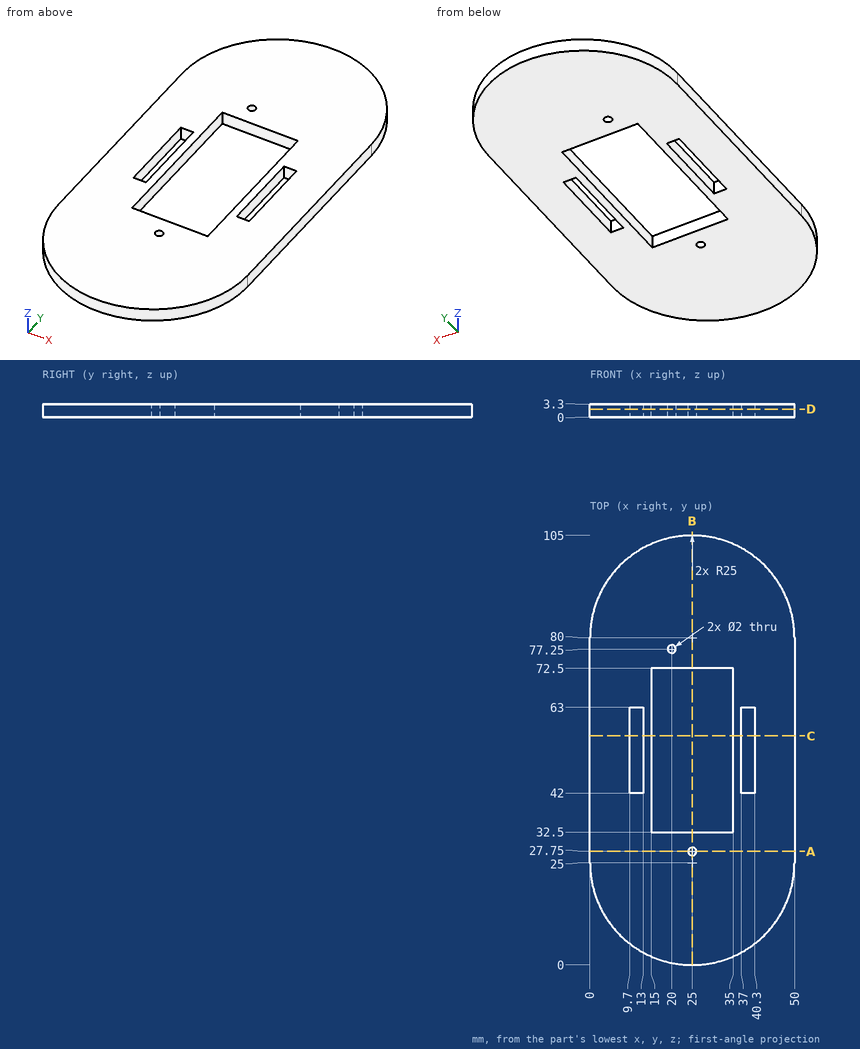
Geometry: see drawing. Coordinates: mm, zero at the bounding-box minimum. Give positions to 0.01 mm unless a question says otherwise; leave off trailing zeros. Order: outer loops, then holes, each group sorted by start corner. A loop starts at its lowest first (then second) coordinate and runs counter-clockwise, first axis right, second up. Notation, with made-up numbers: (-31.75, -5) -> (10.25, -5) arc R21 cw to (10.25, 15) -> close; hole circle Ø9 at (62.25, 85). An arc over 180 degrees is marked (long way). Write each question's results on one line, items separated by ' | '. Start each with the question number.
1) Section B-B (x = 25). Return loops of the section in (y, z).
2) Section A-A (y = 27.75). Return loops of the section in (x, z), then the cut area to 3 significant figures.
3) Section D-D (z = 2.05). Return loops of the section in (x, y).
4) Line query: line 1 (Y direction, x = 20, z = 2.5); line 2 (X direction, y = 57, z = 1.2); line 3 (Y direction, x = 25, z = 3.1). Output: solid intervals per line, ascending. Write a range as from..to.
5) Section C-C (y = 56). Return loops of the section in (x, z), then the cut area to 3 significant figures.
6) First-contact query: pin 1 (1.6 mm diameter, centred on x = 12, z = 1, fed in from +Y); pin 2 (1 mm diameter, centred on x = 11, z = 1, fed in from -Y); pin 3 (1.6 mm diameter, centred on x = 22.5, z = 1.5, fed in from -Y). Flat tips, straight axial feed; report the tip coordinate or a pass-through.
Calculated:
1) outline: (0, 0) -> (26.75, 0) -> (26.75, 3.3) -> (0, 3.3) -> close; (28.75, 0) -> (32.5, 0) -> (32.5, 3.3) -> (28.75, 3.3) -> close; (72.5, 0) -> (105, 0) -> (105, 3.3) -> (72.5, 3.3) -> close
2) outline: (0, 0) -> (24, 0) -> (24, 3.3) -> (0, 3.3) -> close; (26, 0) -> (50, 0) -> (50, 3.3) -> (26, 3.3) -> close | area: 158 mm2
3) outline: (0, 25) arc R25 ccw to (50, 25) -> (50, 80) arc R25 ccw to (0, 80) -> close; hole (9.7, 42) -> (13, 42) -> (13, 63) -> (9.7, 63) -> close; hole (15, 32.5) -> (35, 32.5) -> (35, 72.5) -> (15, 72.5) -> close; hole circle Ø2 at (20, 77.25); hole circle Ø2 at (25, 27.75); hole (37, 42) -> (40.3, 42) -> (40.3, 63) -> (37, 63) -> close
4) line 1: 0.51..32.5, 72.5..76.25, 78.25..104.49 | line 2: 0..9.7, 13..15, 35..37, 40.3..50 | line 3: 0..26.75, 28.75..32.5, 72.5..105
5) outline: (0, 0) -> (9.7, 0) -> (9.7, 3.3) -> (0, 3.3) -> close; (13, 0) -> (15, 0) -> (15, 3.3) -> (13, 3.3) -> close; (35, 0) -> (37, 0) -> (37, 3.3) -> (35, 3.3) -> close; (40.3, 0) -> (50, 0) -> (50, 3.3) -> (40.3, 3.3) -> close | area: 77.2 mm2
6) pin 1: y = 101.82 | pin 2: y = 3.96 | pin 3: y = 0.06
